Design review of the part built by this model. Coordinates are the model's own, in mm. Face numbers are marked on the shaded views. A direction names the side the tool comes from. Round coordinates to 2 decimals unless told otherwise and drop trailing zeros. Order: outer loops, then holes, each group sorted by start corner. A loop starts at its lowest first (then second) coordinate and runs counter-clockwise, first axis right, second up. Notation, with made-up numbers: M 46,78 L 64,78 A12 cw 64,91 Z; hole C 47,37 d7. An arc over 180 degrees is marked long. Use a Markdown table: item, result. Add a question column.
(1) Take a section at B-B (y = 0). Write out the cut boundary in (x, z).
(2) Machinability: for the marked faces 5, 6, 7 and 8, which of the approach directions +Z, -Z, +X, -X, +Y, -Y give a long, thin tool a straight path to every point of the face, cutting with its end or side? Answer none if there is none.
(3) Take a section at C-C (x = 51.5). Write out the cut boundary in (y, z).
(4) To check wall thickness, follow probe 1 along Y at (x, z) = (15.5, 6.25); probe 2 along Z at (x, y) = (19, -17); probe 3 along Y at (x, z) = (-48, 47.5). State the ranges of each line that lie inside material, in increasing order. Write a range as from..to.
(5) For pin 1 (3 mm diameter, centred on x = -10, z = 22.5, fed in from -Y); pin 2 (7.5 mm diameter, centred on x = -37.5, z = 22, fed in from -Y); pin 3 (1 mm diameter, centred on x = -13.5, z = 32, fed in from +Y), all flat-tipped, find the tip position at first contact; note any pin that passes through.
(6) Take a section at D-D (y = -37.5). Write out the cut boundary in (x, z).
(7) The part is to be moulded in two halves that separate along Y. For the marked faces 1, 2, 3 and 4, say which applies: released by +Y, released by -Y, zero draft, split by the parting line, or undercut.
Autodesk Fusion 360 part; units mm, degrees
sketch "Baza" plane through (0, 0, 0) normal (0, 0, 1) x (1, 0, 0)
  line L0 (16.2203, 44) -> (-15.5, 44)
  line L1 (-15.5, -22) -> (-15.5, -44)
  line L2 (-15.5, -44) -> (16.3266, -44)
  circle A0 centre (15.5, 25) radius 5
  circle A1 centre (15.5, -25) radius 5
  line L3 (15.5, 44) -> (51.5, 44) construction
  line L4 (15.5, -44) -> (51.5, -44) construction
  line L5 (51.5, 44) -> (51.5, -44) construction
  line L6 (-40, 0) -> (51.5, 0) construction
  line L7 (15.5, 25) -> (15.5, 20) construction
  line L8 (15.5, -20) -> (15.5, -25) construction
  line L9 (-15.5, 44) -> (-28.5, 44)
  line L10 (-28.5, 44) -> (-28.5, 25)
  line L11 (-28.5, -44) -> (-15.5, -44)
  line L12 (-12.5, -19) -> (-12.4999, -19) construction
  line L13 (-41.2176, -9.5) -> (-41.2176, 9.5) construction
  line L14 (-12.5, 19) -> (-12.4999, 19) construction
  circle A2 centre (-41.2176, 0) radius 9.5
  line L15 (-28.5, -25) -> (-28.5, -44)
  line L16 (-34.5, 19) -> (-41.2176, 19)
  arc A3 (-34.5, 19) -> (-28.5, 25) centre (-34.5, 25) ccw
  line L17 (-34.5, -19) -> (-41.2176, -19)
  arc A4 (-28.5, -25) -> (-34.5, -19) centre (-34.5, -25) ccw
  arc A5 (-41.2176, 19) -> (-41.2176, -19) centre (-41.2176, 0) ccw
  line L18 (-15.5, 44) -> (-15.5, 22)
  arc A6 (-15.5, 22) -> (-12.4999, 19) centre (-12.5, 22) ccw
  arc A7 (-12.4999, -19) -> (-15.5, -22) centre (-12.5, -22) ccw
  line L19 (-12.5, 4.9885) -> (-8.5, 4.9885)
  line L20 (-8.5, 4.9885) -> (-8.5, -5.0115)
  line L21 (-8.5, -5.0115) -> (-12.5, -5.0115)
  line L22 (-12.5, 19) -> (-12.5, 4.9885)
  line L23 (-12.5, -5.0115) -> (-12.5, -19)
  line L24 (64.6465, -13.1465) -> (64.935, -13.435) construction
  line L25 (51.5, 0) -> (70.5, 0) construction
  line L26 (64.6437, 13.1437) -> (64.935, 13.435) construction
  line L27 (61.6515, 15.6805) -> (23.5586, 41.7307)
  line L28 (61.6703, -15.6734) -> (23.6778, -41.7219)
  arc A8 (16.3266, -44) -> (23.6778, -41.7219) centre (16.3266, -31) ccw
  arc A9 (23.5586, 41.7307) -> (16.2203, 44) centre (16.2203, 31) ccw
  arc A10 (61.6703, -15.6734) -> (61.6515, 15.6805) centre (50.9262, -0.0029) ccw
  dimension "d1" = 88
  dimension "d2" = 31
  dimension "d3" = 50
  dimension "d5" = 10
  dimension "d6" = 10
  dimension "d7" = 36
  dimension "d12" = 13
  dimension "d13" = 38
  dimension "d15" = 3
  dimension "d16" = 19
  dimension "d18" = 6
  dimension "d20" = 6
  dimension "d21" = 3
  dimension "d22" = 3
  dimension "d23" = 10
  dimension "d24" = 20
  dimension "d27" = 13
  dimension "d28" = 13
  dimension "d29" = 19
extrude "Extrude1" add sketch "Baza" along normal blind 50 contours L1 L9 L10 L11 L15 L16 A3 L17 A4 A5 L18 A6 A7 L19 L20 L21 L22 L23
extrude "Extrude2" add sketch "Baza" along normal blind 10 contours L0 L1 L2 L18 A6 A7 L19 L20 L21 L22 L23 L27 L28 A8 A9 A10
sketch "Triunghi" plane through (0, 0, 0) normal (0, 1, 0) x (1, 0, 0)
  line L0 (-8.5, -50) -> (-8.5, -10)
  line L1 (-8.5, -10) -> (58.5, -10)
  line L2 (-15.5, 0) -> (16.3266, 0)
  line L3 (-15.5, -10) -> (-15.5, -50)
  line L4 (-8.5, -50) -> (58.5, -10)
  dimension "d34" = 10
  dimension "d41" = 40
  dimension "d42" = 67
extrude "Extrude3" add sketch "Triunghi" along normal mid plane 10
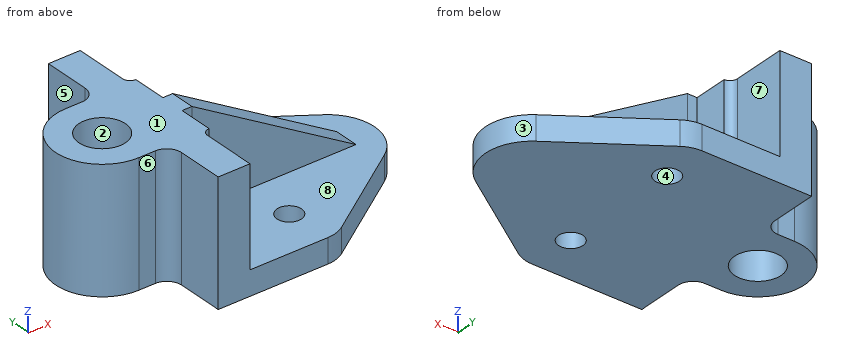
Verdict:
| question | item | result |
|---|---|---|
| 1 | outline | M -60.22,0 L -50.72,0 L -50.72,50 L -60.22,50 Z; M -31.72,0 L 69.93,0 L 69.93,10 L 58.5,10 L -8.5,50 L -31.72,50 Z |
| 2 | face 5 | +Z, -Z, -X, +Y |
| 2 | face 6 | +Z, -Z, -X, -Y |
| 2 | face 7 | +Z, +X, +Y |
| 2 | face 8 | +Z, +X |
| 3 | outline | M -22.65,0 L 22.62,0 L 22.62,10 L 5,10 L 5,14.18 L -5,14.18 L -5,10 L -22.65,10 Z |
| 4 | probe 1 | y = -44..-30, -20..20, 30..44 |
| 4 | probe 2 | z = 0..10 |
| 4 | probe 3 | y = -17.75..-6.65, 6.65..17.75 |
| 5 | pin 1 | stops at y = -5.01 |
| 5 | pin 2 | stops at y = -19.05 |
| 5 | pin 3 | stops at y = 19.4 |
| 6 | outline | M -28.5,0 L 29.84,0 L 29.84,10 L -15.5,10 L -15.5,50 L -28.5,50 Z |
| 7 | face 1 | zero draft |
| 7 | face 2 | undercut |
| 7 | face 3 | split by the parting line |
| 7 | face 4 | undercut |
